Could you check a few things on this drawing? It's one solid part, dimensions in mm from its lowest x, y, z. A direction names the side the tool comes from. Give positions to 0.01 mm unless a question says otherwise; leave off trailing zeros. Loops run counter-clockwise (first coordinate to the right, second up) from the corner with the lowest first, then second, coordinate; pieces in that order, holes last.
Q1. For the marked faces 1 and 2, which set-ups out of +Z, -Z, +X, -X, +Y, -Y let a thin tool reach every point of the face, with its end or its side?
Q2. Suppose I cut it at C-C (y = 28.25). List the corners of the cut face in (x, z) for me, and give its area (3 significant figures).
Q3. Suppose I cut it at D-D (x = 14). List the corners of the cut face in (y, z) for me, and give its area (3 significant figures).
Q4. Thinking about a two-plate mould opening in Z: for the marked faces 3, 4 and 5, which applies, pulls with the +Z half, pulls with the -Z half, needs draft (parallel to the pull), parting line crosses it, or undercut?
Q5. Suppose I cut it at B-B (z = 19). List the corners of the cut face in (x, y) for me, and give its area (3 significant figures).
Q6. I need wall thicknesses on probe 1 along X at (y, z) = (10.75, 14.5); probe 2 along Z at (x, y) = (35.5, 13.25); probe 3 along Y at (x, z) = (35, 28.5). Which ranges of each line are inside material? Lowest first, please.
Q7. Suppose I cut it at A-A (z = 12.5). List the corners of the cut face in (x, y) for me, and give its area (3 significant figures).
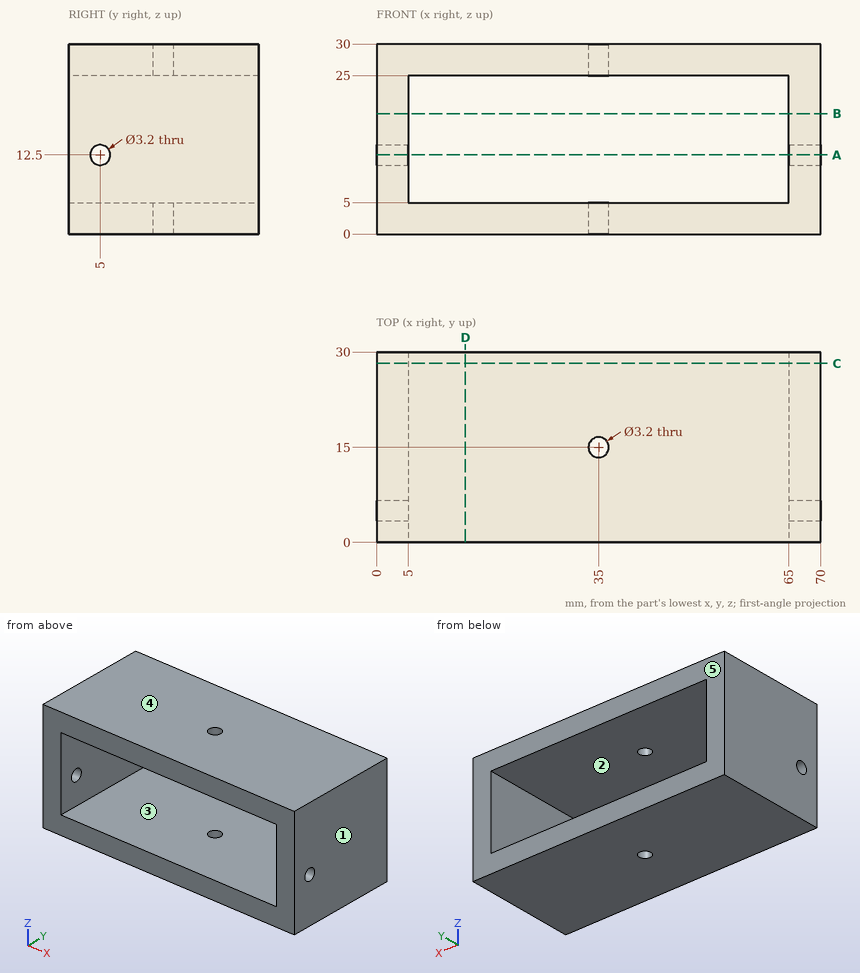
Solutions:
1. face 1: +Z, -Z, +X, +Y, -Y
1. face 2: +Y, -Y
2. outline: (0, 0) - (70, 0) - (70, 30) - (0, 30) - close; hole (5, 5) - (65, 5) - (65, 25) - (5, 25) - close
2. area: 900 mm2
3. outline: (0, 0) - (30, 0) - (30, 5) - (0, 5) - close; (0, 25) - (30, 25) - (30, 30) - (0, 30) - close
3. area: 300 mm2
4. face 3: undercut
4. face 4: pulls with the +Z half
4. face 5: needs draft
5. outline: (0, 0) - (5, 0) - (5, 30) - (0, 30) - close; (65, 0) - (70, 0) - (70, 30) - (65, 30) - close
5. area: 300 mm2
6. probe 1: x = 0 to 5, 65 to 70
6. probe 2: z = 0 to 5, 25 to 30
6. probe 3: y = 0 to 13.4, 16.6 to 30
7. outline: (0, 0) - (5, 0) - (5, 3.4) - (0, 3.4) - close; (0, 6.6) - (5, 6.6) - (5, 30) - (0, 30) - close; (65, 0) - (70, 0) - (70, 3.4) - (65, 3.4) - close; (65, 6.6) - (70, 6.6) - (70, 30) - (65, 30) - close
7. area: 268 mm2
